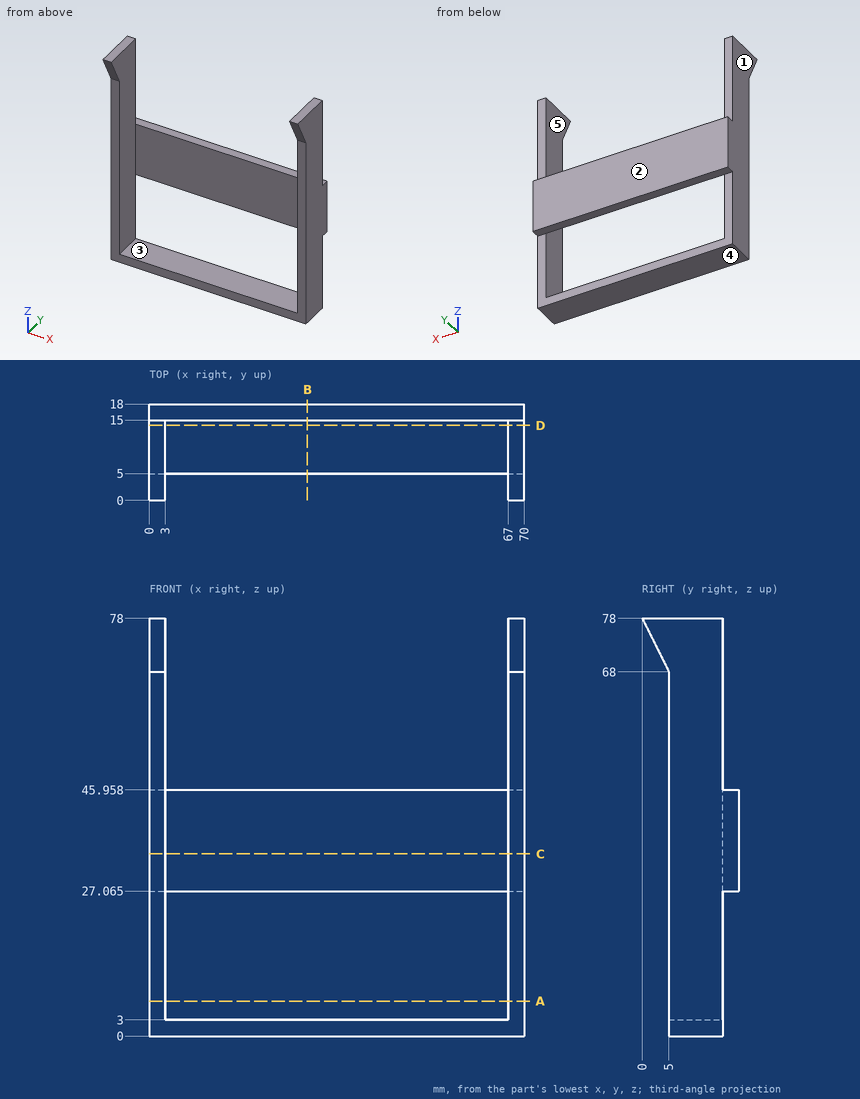
Input: dimensioned drawing with shaded views. Units: mm. Origin: part minimum x, y, z. A direction names the side the tool comes from. Round coordinates to 2 decimals unless told otherwise and drop trailing zeros. Order: outer loops, then holes, each group sorted by start corner. A loop starts at its lowest first (then second) coordinate and runs counter-clockwise, first axis right, second up.
Q1. Mould query, pull axis X, two halves, no side actions, for the marked faces 1, 2 and 3. Classes: released by +X, released by -X, zero draft, split by the parting line, or undercut.
Result sheet:
face 1: released by -X
face 2: zero draft
face 3: undercut
Q2. Material intervals for probe 1 along X at (y, z) = (11, 10); probe 2 along Z at (x, y) = (42, 6.75); probe 3 along Y at (x, z) = (22.5, 32.5), sorted ascending.
Result sheet:
probe 1: x = 0 to 3, 67 to 70
probe 2: z = 0 to 3
probe 3: y = 15 to 18
Q3. Pin query (flat end, axial travel): pin 1 (1.5 mm diameter, centred on x = 46.5, y = 16, fed in from +Z); pin 2 (2.5 mm diameter, centred on x = 22, y = 16.5, fed in from -Z) (1 decimal); pin 3 (1.5 mm diameter, centred on x = 1, z = 68, fed in from +Y). Return the tip coordinate at first contact, or that it passes through.
Result sheet:
pin 1: stops at z = 45.96
pin 2: stops at z = 27.1
pin 3: stops at y = 15
Q4. Access query for the marked faces 4 and 5. Directions: +Z, -Z, +X, -X, +Y, -Y. A direction counts if a zero-diameter tool reaches every point of the face in a straight line with its end or side. Return the directions, or none.
Result sheet:
face 4: -Z, +X, -X, +Y, -Y
face 5: +Z, -Y
Q5. Section B-B, the plane x = 29.5. Output: boundary loops of the cut face in (y, z) (1 decimal).
Result sheet:
outline: (5, 0) - (15, 0) - (15, 3) - (5, 3) - close; (15, 27.1) - (18, 27.1) - (18, 46) - (15, 46) - close
Q6. Section A-A, the plane z = 6.5. Output: boundary loops of the cut face in (x, y).
Result sheet:
outline: (0, 5) - (3, 5) - (3, 15) - (0, 15) - close; (67, 5) - (70, 5) - (70, 15) - (67, 15) - close
Q7. Section D-D, the plane y = 14. Output: boundary loops of the cut face in (x, z), and give its area (3 significant figures).
Result sheet:
outline: (0, 0) - (70, 0) - (70, 78) - (67, 78) - (67, 3) - (3, 3) - (3, 78) - (0, 78) - close
area: 660 mm2
Q8. Section C-C, the plane z = 34. Output: boundary loops of the cut face in (x, y), and give its area (3 significant figures).
Result sheet:
outline: (0, 5) - (3, 5) - (3, 15) - (67, 15) - (67, 5) - (70, 5) - (70, 18) - (0, 18) - close
area: 270 mm2
